from build123d import *

# Parameters (mm, degrees)
BOSS_EXTRUDE1_DEPTH     = 100
SKETCH2_R               = 10
BOSS_EXTRUDE2_DEPTH     = 67
SKETCH3_R               = 6
CUT_EXTRUDE1_DEPTH      = 67
SKETCH4_R               = 6
CUT_EXTRUDE2_DEPTH      = 67
CUT_EXTRUDE2_DEPTH_BACK = 67
BOSS_EXTRUDE3_DEPTH     = 3
SKETCH9_W               = 6.067764808
SKETCH9_H               = 8.847787213
BOSS_EXTRUDE4_DEPTH     = 26.5
CUT_EXTRUDE3_DEPTH      = 26.5
SKETCH11_W              = 5.758839732
SKETCH11_H              = 8.847787213
BOSS_EXTRUDE5_DEPTH     = 42
CUT_EXTRUDE4_DEPTH      = 42
SKETCH13_W              = 1.235315599
SKETCH13_H              = 5.758839732
CUT_EXTRUDE6_DEPTH      = 42


with BuildPart() as part:
    # Sketch1 → Boss-Extrude1 (new body)
    with BuildSketch(Plane.XY):
        Polygon((-61.723716381, 0), (-27.5, 0), (-27.5, 9.902200489), (27.5, 9.902200489), (27.5, 0), (73.276283619, 0), (73.276283619, 9.902200489), (31.668314846, 9.902200489), (31.668314846, 18.749987702), (-34.880531234, 18.749987702), (-34.880531234, 9.902200489), (-61.723716381, 9.902200489), align=None)
    extrude(amount=-BOSS_EXTRUDE1_DEPTH)

    # Sketch2 → Boss-Extrude2 (add)
    with BuildSketch(Plane.ZY.offset(34.880531234)):
        with BuildLine():
            Line((-100, 9.902200489), (-100, 54.908843962))
            ThreePointArc((-100, 54.908843962), (-81.480595065, 67.356914351), (-62.96119013, 54.908843962))
            Line((-62.96119013, 54.908843962), (-62.96119013, 18.749987702))
            Line((-62.96119013, 18.749987702), (0, 18.749987702))
            Line((0, 18.749987702), (0, 9.902200489))
            Line((0, 9.902200489), (-100, 9.902200489))
        make_face()
        with Locations((-81.480595065, 47.356914351)):
            Circle(SKETCH2_R, mode=Mode.SUBTRACT)
    extrude(amount=-BOSS_EXTRUDE2_DEPTH)

    # Sketch3 → Cut-Extrude1 (cut)
    with BuildSketch(Plane(origin=(0, 9.902200489, 0), x_dir=(1, 0, 0), z_dir=(0, 1, 0))):
        with Locations((-48.302123808, 24.983488629)):
            Circle(SKETCH3_R)
        with Locations((-48.302123808, 75.004643802)):
            Circle(SKETCH3_R)
    extrude(amount=-CUT_EXTRUDE1_DEPTH, mode=Mode.SUBTRACT)

    # Sketch4 → Cut-Extrude2 (cut, two sides)
    with BuildSketch(Plane(origin=(0, 0, 0), x_dir=(1, 0, 0), z_dir=(0, 1, 0))) as cut_extrude2_sk:
        with Locations((57.109031968, 75.004643802)):
            Circle(SKETCH4_R)
        with Locations((57.109031968, 24.983488629)):
            Circle(SKETCH4_R)
    extrude(amount=CUT_EXTRUDE2_DEPTH, mode=Mode.SUBTRACT)
    extrude(cut_extrude2_sk.sketch, amount=-CUT_EXTRUDE2_DEPTH_BACK, mode=Mode.SUBTRACT)

    # Sketch5 → Boss-Extrude3 (add, symmetric)
    with BuildSketch(Plane(origin=(0, 0, 0), x_dir=(0, 0, -1), z_dir=(1, 0, 0))):
        Polygon((62.96119013, 54.908843962), (0, 18.749987702), (62.96119013, 18.749987702), align=None)
    extrude(amount=BOSS_EXTRUDE3_DEPTH, both=True)

    # Sketch9 → Boss-Extrude4 (add)
    with BuildSketch(Plane.ZY.offset(34.880531234)):
        with Locations((-47.773735316, 14.326094096)):
            Rectangle(SKETCH9_W, SKETCH9_H)
    extrude(amount=BOSS_EXTRUDE4_DEPTH)

    # Sketch10 → Cut-Extrude3 (cut)
    with BuildSketch(Plane.XY.offset(-44.739852912)):
        Polygon((-34.880531234, 18.749987702), (-61.380531234, 10), (-61.380531234, 18.749987702), align=None)
    extrude(amount=-CUT_EXTRUDE3_DEPTH, mode=Mode.SUBTRACT)

    # Sketch11 → Boss-Extrude5 (add)
    with BuildSketch(Plane(origin=(32.119468766, 0, 0), x_dir=(0, 0, -1), z_dir=(1, 0, 0))):
        with Locations((48.947532941, 14.326094096)):
            Rectangle(SKETCH11_W, SKETCH11_H)
    extrude(amount=BOSS_EXTRUDE5_DEPTH)

    # Sketch12 → Cut-Extrude4 (cut)
    with BuildSketch(Plane(origin=(0, 0, -51.826952807), x_dir=(-1, 0, 0), z_dir=(0, 0, -1))):
        Polygon((-32.119468766, 18.749987702), (-72.884153167, 10), (-74.975846316, 10), (-74.119468766, 18.749987702), align=None)
    extrude(amount=-CUT_EXTRUDE4_DEPTH, mode=Mode.SUBTRACT)

    # Sketch13 → Cut-Extrude6 (cut)
    with BuildSketch(Plane(origin=(0, 10, 0), x_dir=(1, 0, 0), z_dir=(0, 1, 0))):
        with Locations((73.501810967, 48.947532941)):
            Rectangle(SKETCH13_W, SKETCH13_H)
    extrude(amount=-CUT_EXTRUDE6_DEPTH, mode=Mode.SUBTRACT)


solid = part.part
Could you check a few things on this model? Use its own coordinates, in mm. A direction names the side the tool comes from. Give positions to 0.01 mm unless a question says otherwise; leave off trailing zeros. Order: outer loops, then holes, each group sorted by start corner. A loop starts at its lowest first (then second) coordinate and runs counter-clockwise, first axis right, second up. Notation, with made-up numbers: (-21.75, 75.25) -> (1.25, 75.25) arc R7 ccw to (1.25, 87.25) -> close; hole circle Ø1 at (11, 67.5). An arc over 180 degrees is marked (long way). Return JSON: item names as keys, results as strings.
1. Imagine slicing it at A-A on x = 58. List the corners of the cut face in (y, z) for me, then the cut area to 3 significant figures.
Answer list:
{"outline": "(0, -100) -> (9.9, -100) -> (9.9, -80.94) -> (0, -80.94) -> close; (0, -69.07) -> (9.9, -69.07) -> (9.9, -51.83) -> (13.19, -51.83) -> (13.19, -46.07) -> (9.9, -46.07) -> (9.9, -30.92) -> (0, -30.92) -> close; (0, -19.05) -> (9.9, -19.05) -> (9.9, 0) -> (0, 0) -> close", "area": "774 mm2"}
2. I need wall thicknesses on line 1 (Z direction, x = 28.5, y = 47.5); line 2 (Z direction, x = 24.5, y = 25); line 3 (X direction, y = 8, z = -71.5). Which ranges of each line are inside material? Lowest first, please. Write a range as from..to.
Answer list:
{"line 1": "z = -100..-91.48, -71.48..-62.96", "line 2": "z = -100..-62.96", "line 3": "x = -61.72..-53.17, -43.43..-27.5, 27.5..52.24, 61.98..73.28"}
3. For pin 1 Ø2 at (y, z) = (50.5, -67.5) entering from -X; pin 2 Ø9.5 at (x, y) = (-25, 34.5) entering from +Z; pin 3 Ø10 at (x, z) = (6, -59) entering from +Y; pin 4 Ø12 at (x, y) = (-43.5, 56) entering from +Z, each with a flat end and sliding along its axis, tell me the tip position at first contact or that it passes through.
Answer list:
{"pin 1": "stops at x = -34.88", "pin 2": "stops at z = -62.96", "pin 3": "stops at y = 57.07", "pin 4": "passes through"}
4. Imagine slicing it at D-D on x = 23. List the corners of the cut face in (y, z) for me, then the cut area to 3 significant figures.
Answer list:
{"outline": "(9.9, -100) -> (54.91, -100) arc R20 ccw to (54.91, -62.96) -> (18.75, -62.96) -> (18.75, 0) -> (9.9, 0) -> close; hole circle Ø20 at (47.36, -81.48)", "area": "2,240 mm2"}
5. Imagine slicing it at C-C on z = -26.5. List the corners of the cut face in (x, y) for me, then the cut area to 3 significant figures.
Answer list:
{"outline": "(-61.72, 0) -> (-54.11, 0) -> (-54.11, 9.9) -> (-61.72, 9.9) -> close; (-42.5, 0) -> (-27.5, 0) -> (-27.5, 9.9) -> (27.5, 9.9) -> (27.5, 0) -> (51.3, 0) -> (51.3, 9.9) -> (32.12, 9.9) -> (32.12, 18.75) -> (3, 18.75) -> (3, 33.97) -> (-3, 33.97) -> (-3, 18.75) -> (-34.88, 18.75) -> (-34.88, 9.9) -> (-42.5, 9.9) -> close; (62.91, 0) -> (73.28, 0) -> (73.28, 9.9) -> (62.91, 9.9) -> close", "area": "1,250 mm2"}
6. Imagine slicing it at B-B on y = 49. List the corners of the cut face in (x, z) for me, then the cut area to 3 significant figures.
Answer list:
{"outline": "(-34.88, -100) -> (32.12, -100) -> (32.12, -91.34) -> (-34.88, -91.34) -> close; (-34.88, -71.62) -> (32.12, -71.62) -> (32.12, -62.96) -> (3, -62.96) -> (3, -52.67) -> (-3, -52.67) -> (-3, -62.96) -> (-34.88, -62.96) -> close", "area": "1,220 mm2"}
7. Thinking about a two-plate mould opening in X: for faces 1 (the flat face through (73.276, 5, -76)), 2 (the flat face through (-27.5, 5, -49)), 3 (the flat face through (-45, 13, -50.808)), which applies, pulls with the +X half, pulls with the -X half, needs draft (parallel to the pull), parting line crosses it, or undercut?
Answer list:
{"face 1": "pulls with the +X half", "face 2": "undercut", "face 3": "needs draft"}
8. On a 3-axis mill with a long thin cutter (end or side, diameter ignored), from which of +Z, -Z, +X, -X, +Y, -Y can I reach the whole of each face in a straight line? I mean faces 4 (the flat face through (-48, 9.902, -38)), 5 (the flat face through (-19, 37, -62.961)), 6 (the flat face through (-34.881, 33, -81)), 7 (the flat face through (48, 9.902, -76)), 8 (the flat face through (3, 29, -45)). Say none if no direction works.
Answer list:
{"face 4": "-X, +Y", "face 5": "+Z, -X, +Y", "face 6": "-Z, -X, +Y", "face 7": "-Z, +X, +Y", "face 8": "+Z, +X, +Y"}
